Could you check a few things on this drawing? It's one solid part, dimensions in mm from its lowest x, y, z. Give positions to 0.01 mm unless a question says otherwise; leave off trailing zeros. Loops run counter-clockwise (first coordinate to the right, second up) from the corner with the lowest first, then second, coordinate; pieces in that order, holes last. Notation, with made-up numbers: (0.25, 34.25) - (27.25, 34.25) arc R15 ccw to (27.25, 60.25) - close; hole circle Ø6 at (88, 79). An arc over 180 degrees is marked (long way). Put each result on its own line as item: value. Start each with the question number.
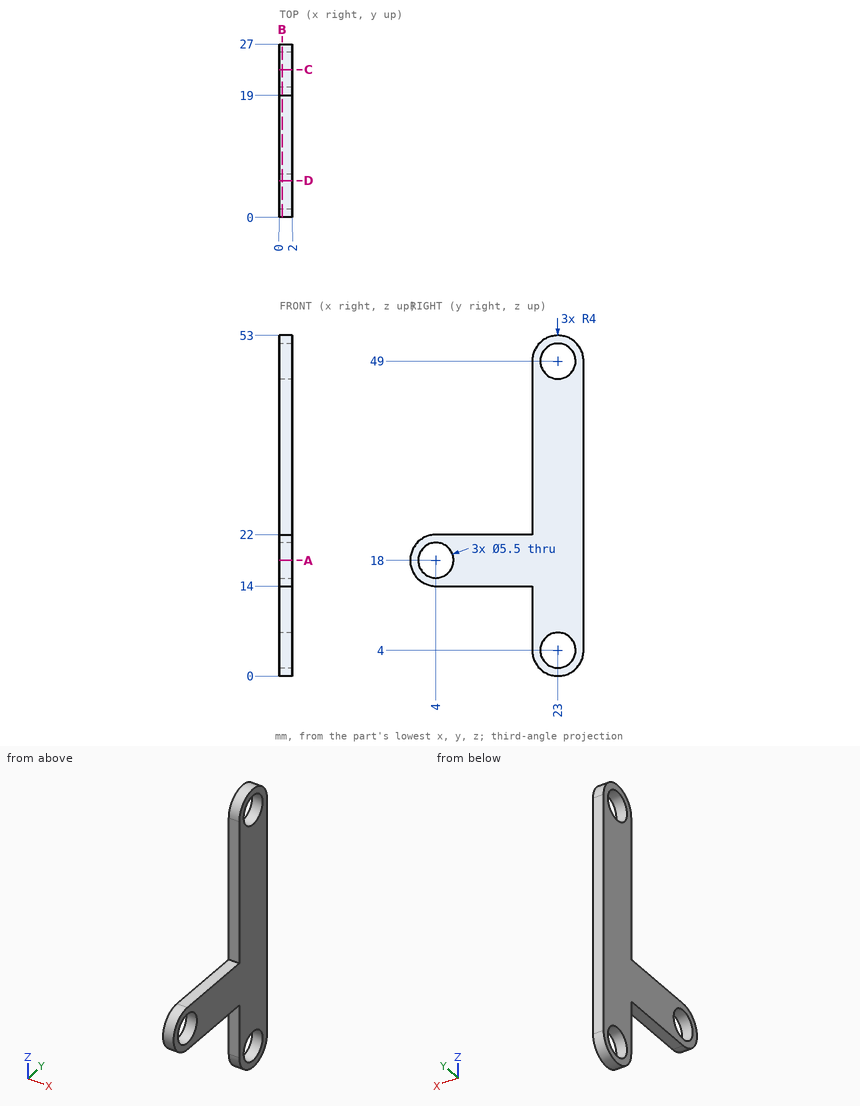
1) I'm going to push flat-ended pins straight in: P1, Ø0.6, axis at x = 1, y = 10.5, coming from the +Z side; P2, Ø1, axis at x = 1.5, y = 3.5, coming from the -Z side; P3, Ø6.5, axis at y = 4, z = 18, coming from the +X side. Where does each tip first touch, or does it pass through?
2) Suppose I cut it at A-A on z = 18. Please give me the cut outline in (x, y), plus the area to 3 significant figures.
3) I need wall thicknesses on line 1 (Y direction, x = 1.4, z = 49); line 2 (Y direction, x = 1.45, z = 41.5); line 3 (Z direction, x = 0.75, y = 24.5). Which ranges of each line are inside material? Lowest first, please.
4) Suppose I cut it at C-C on y = 23. Please give me the cut outline in (x, z).
5) Suppose I cut it at B-B on x = 0.45. Please give me the cut outline in (y, z).
6) Suppose I cut it at D-D on y = 5.75. Please give me the cut outline in (x, z).
Ans:
1. P1: stops at z = 22
1. P2: stops at z = 14
1. P3: stops at x = 2
2. outline: (0, 0) - (2, 0) - (2, 1.25) - (0, 1.25) - close; (0, 6.75) - (2, 6.75) - (2, 27) - (0, 27) - close
2. area: 43.0 mm²
3. line 1: y = 19 to 20.25, 25.75 to 27
3. line 2: y = 19 to 27
3. line 3: z = 0.29 to 1.7, 6.3 to 46.7, 51.3 to 52.71
4. outline: (0, 0) - (2, 0) - (2, 1.25) - (0, 1.25) - close; (0, 6.75) - (2, 6.75) - (2, 46.25) - (0, 46.25) - close; (0, 51.75) - (2, 51.75) - (2, 53) - (0, 53) - close
5. outline: (4, 14) - (19, 14) - (19, 4) arc R4 ccw to (27, 4) - (27, 49) arc R4 ccw to (19, 49) - (19, 22) - (4, 22) arc R4 ccw to start; hole circle Ø5.5 at (4, 18); hole circle Ø5.5 at (23, 4); hole circle Ø5.5 at (23, 49)
6. outline: (0, 14) - (2, 14) - (2, 15.88) - (0, 15.88) - close; (0, 20.12) - (2, 20.12) - (2, 22) - (0, 22) - close
